Autodesk Inventor part; units mm, degrees
ref_plane "YZ Plane" through (0, 0, 0) normal (1, 0, 0) x (0, 1, 0)
ref_plane "XZ Plane" through (0, 0, 0) normal (0, 1, 0) x (-1, 0, 0)
ref_plane "XY Plane" through (0, 0, 0) normal (0, 0, 1) x (1, 0, 0)
sketch "スケッチ1" plane through (0, 0, 0) normal (0, 0, 1) x (1, 0, 0)
  arc A0 (0.7632, 11.9121) -> (-1.0179, 11.893) centre (0, 0) ccw construction
  arc A1 (0.4062, 11.3607) -> (-0.4062, 11.3607) centre (0, 0) ccw
  arc A2 (9.3048, 1.5803) -> (-9.0567, 2.6555) centre (0, 0) ccw construction
  arc A3 (0.8923, 10.7753) -> (1.9623, 9.2318) centre (2.2471, 10.5718) ccw
  line L0 (1.9623, 9.2318) -> (0, 0)
  arc A4 (-1.9623, 9.2318) -> (-0.8923, 10.7753) centre (-2.2471, 10.5718) ccw
  line L1 (-1.9623, 9.2318) -> (0, 0)
  arc A5 (-0.4062, 11.3607) -> (-0.8923, 10.7753) centre (-0.388, 10.8511) ccw
  arc A6 (0.8923, 10.7753) -> (0.4062, 11.3607) centre (0.388, 10.8511) ccw
  line L2 (0, 0) -> (0, 2.9942) construction
  dimension "d0" = 11.9365
  dimension "d1" = 11.368
  dimension "d2" = 1.93
  dimension "d3" = 0.51
  dimension "d4" = 1.37
  dimension "d5" = 1.37
  dimension "d6" = 24
  dimension "d7" = 12
extrude "押し出し1" add sketch "スケッチ1" along normal blind 5
pattern_circular "円形状パターン1" count 15 over 360 about axis through (0, 0, 0) along (0, 0, 1) of "押し出し1"
sketch "スケッチ2" plane through (0, 0, 5) normal (0, 0, 1) x (1, 0, 0)
  circle A0 centre (0, 0) radius 14
  dimension "d13" = 28
extrude "押し出し2" add sketch "スケッチ2" along normal blind 1
sketch "スケッチ3" plane through (0, 0, 0) normal (0, 0, -1) x (-1, 0, 0)
  circle A0 centre (0, 0) radius 4
  circle A1 centre (0, 7) radius 1.25
  circle A2 centre (-7, 0) radius 1.25
  circle A3 centre (7, 0) radius 1.25
  dimension "d16" = 8
  dimension "d18" = 2.5
  dimension "d19" = 7
  dimension "d20" = 2.5
  dimension "d21" = 2.5
  dimension "d22" = 7
  dimension "d23" = 7
extrude "押し出し3" cut sketch "スケッチ3" against normal through all
properties part number "プーリ_歯数15_2.5mm" material "アセタール樹脂、白"
Could you check a few things on this model? Use its own coordinates, in mm. A direction names the side the tool comes from. Give positions to 0.01 mm unless a question says otherwise; leave off trailing zeros. Return JSON: item names as keys, results as strings.
Item 1: I need wall thicknesses on L1, parallel to Y at x = 0, z = 1.95; L2, parallel to Y at x = 7, z = 3.6; L3, parallel to X at y = -0.75, z = 3.7. Which ranges of each line are inside material? Lowest first, please. Write a range as from..to.
Geometry results:
{"L1": "y = -9.44..-4, 4..5.75, 8.25..11.37", "L2": "y = -8.96..-8.13, -6.33..-1.25, 1.25..7.54", "L3": "x = -11.34..-8, -6..-3.93, 3.93..6, 8..11.34"}
Item 2: Which directions (+Z, -Z, +X, -X, +Y, -Y) give clear straight access to the entire face, cutting with the end or side of a thin tool? Please do faces 5 (the cylindrical face through (-6.662, -7.248, 2.465)), 6 (the cylindrical face through (-1, 10, 2)), 7 (the cylindrical face through (-6.512, 7.383, 2.465)), 8 (the cylindrical face through (8.023, 5.704, 2.465)).
Geometry results:
{"face 5": "-Z, -X", "face 6": "-Z", "face 7": "-Z, +Y", "face 8": "-Z, +X"}
Item 3: If we section it at A-A on z = 3.7: Count the separate pieces of the cut face and the enclosed holes in it, plus the area to 3 significant figures.
Geometry results:
{"separate pieces": "1", "enclosed holes": "4", "area": "273 mm²"}
Item 4: We'd pull the mould along Y, two halves only. Please class faces 1 (the cylindrical face through (-3.14, -9.33, 2.46)), 2 (the cylindrical face through (4.834, -8.576, 2.465)), 3 (the cylindrical face through (-9.844, 0.101, 2.465)), 4 (the cylindrical face through (-0.006, 11.368, 2.465)): +Y half, -Y half, draft (parallel to the pull), parting line (faces both ways), or undercut.
Geometry results:
{"face 1": "undercut", "face 2": "-Y half", "face 3": "undercut", "face 4": "+Y half"}
Item 5: I'm going to push flat-ended pins straight in: pin 1 (1.5 mm diameter, centred on x = -7, y = 0, fed in from +Z); pin 2 (1 mm diameter, centred on y = 8, z = 2.5, fed in from -X); pin 3 (1 mm diameter, centred on y = -1.5, z = 5.5, fed in from +X). Where does each tip first touch, or does it pass through?
Geometry results:
{"pin 1": "passes through", "pin 2": "stops at x = -8.54", "pin 3": "stops at x = 13.96"}
